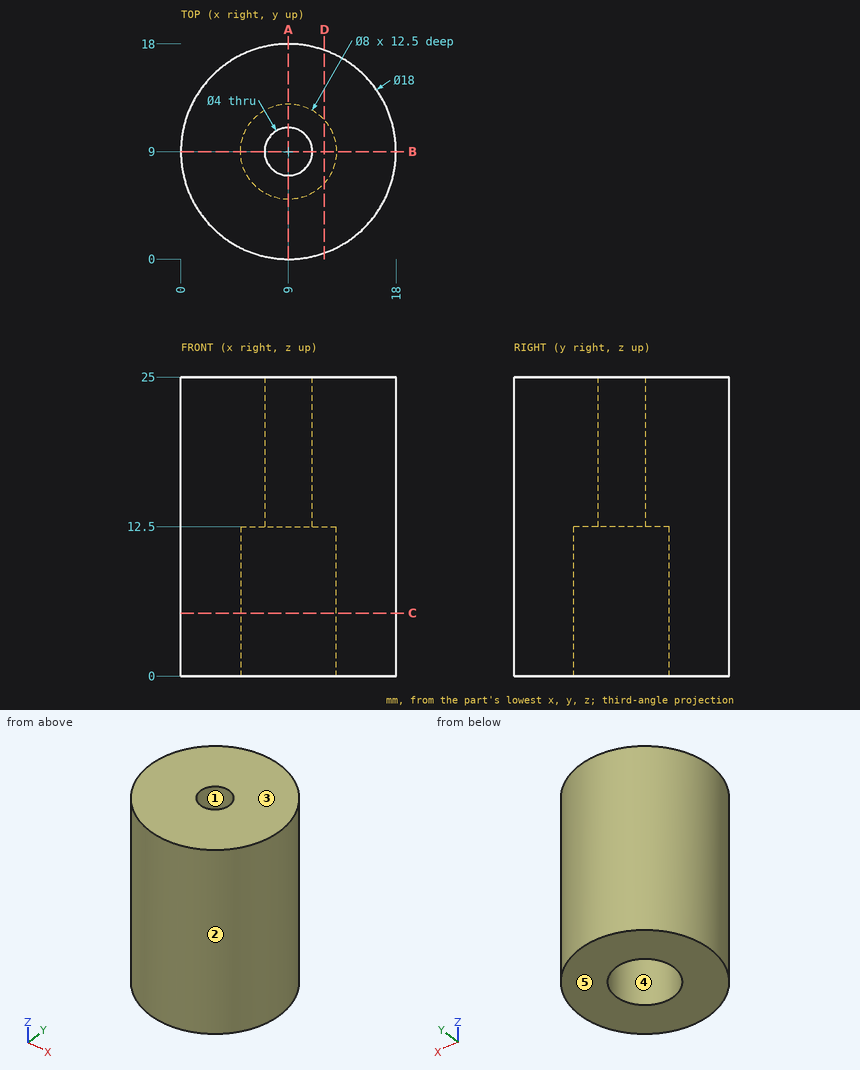
Study the drawing (mm; zero at the part's minimum x, y, z) and answer. A direction names the side the tool comes from. Give positions to 0.01 mm unless a question says otherwise; leave off trailing zeros. Loops run counter-clockwise (first coordinate to the right, second up) from the corner with the lowest first, then second, coordinate; pieces in that order, holes last. Notation, with made-up numbers: (4.5, 7) - (21.5, 7) arc R15 cw to (21.5, 22) - close; hole circle Ø2 at (82, 37.25). An arc over 180 degrees is marked (long way). Return JSON: item names as keys, results as strings. Group by question number.
1. Find section D-D (x = 12). Write down the section's boundary in (y, z).
2. Determine the mould class of the marked faces 1, 2 and 3 for opening direction X: pulls with the +X half, pulls with the -X half, needs draft (parallel to the pull), parting line crosses it, or undercut.
3. Find section C-C (z = 5.25). Write down the section's boundary in (x, y).
4. Given pin 1 Ø9 at (x, y) = (9, 9) entering from +Z; pin 2 Ø3 at (y, z) = (15, 22) entering from -X; pin 3 Ø1.5 at (y, z) = (13.5, 17) entering from +X; pin 4 Ø1.5 at (y, z) = (15, 11) entering from +X, each flat-ended and moving along its own axis, determine where each tip first touches the part or whether it passes through.
5. Find section A-A (x = 9). Write down the section's boundary in (y, z).
6. Which of the six approach directions +Z, -Z, +X, -X, +Y, -Y give full straight-line access (tool end or side, diameter ignored) to the marked faces 4 and 5?
7. Straight lines are drawn through the part: line 1 (Y direction, x = 9, z = 16); line 2 (Y direction, x = 10.5, z = 6.5); line 3 (Z direction, x = 9, y = 11.75). For each, find the intervals that lie inside material, in ascending order. Write a range as [from, to].
Verdict:
{
 "1": {"outline": "(0.51, 0) - (6.35, 0) - (6.35, 12.5) - (11.65, 12.5) - (11.65, 0) - (17.49, 0) - (17.49, 25) - (0.51, 25) - close"},
 "2": {"face 1": "undercut", "face 2": "parting line crosses it", "face 3": "needs draft"},
 "3": {"outline": "circle Ø18 at (9, 9); hole circle Ø8 at (9, 9)"},
 "4": {"pin 1": "stops at z = 25", "pin 2": "stops at x = 1.21", "pin 3": "stops at x = 17.18", "pin 4": "stops at x = 16.31"},
 "5": {"outline": "(0, 0) - (5, 0) - (5, 12.5) - (7, 12.5) - (7, 25) - (0, 25) - close; (11, 12.5) - (13, 12.5) - (13, 0) - (18, 0) - (18, 25) - (11, 25) - close"},
 "6": {"face 4": "-Z", "face 5": "-Z, +X, -X, +Y, -Y"},
 "7": {"line 1": "y = [0, 7], [11, 18]", "line 2": "y = [0.13, 5.29], [12.71, 17.87]", "line 3": "z = [12.5, 25]"}
}
